```python
from build123d import *

# Parameters (mm, degrees)
BOSS_EXTRUDE1_DEPTH              = 6.35
F_17_64_0_26563_DIAMETER_HOLE1_D = 6.747002
FILLET1_R                        = 6.35
F_10_0_1935_DIAMETER_HOLE1_D     = 4.9149
SKETCH8_R                        = 3.373501
CUT_EXTRUDE1_DEPTH               = 299.268395545
FILLET2_R                        = 12.7


with BuildPart() as part:
    # Sketch1 → Boss-Extrude1 (new body)
    with BuildSketch(Plane(origin=(0, 0, 0), x_dir=(1, 0, 0), z_dir=(0, 1, 0))):
        with BuildLine():
            Line((-268.2875, -15.875), (-233.3625, -15.875))
            ThreePointArc((-233.3625, -15.875), (-228.872371939, -17.734871939), (-227.0125, -22.225))
            Line((-227.0125, -22.225), (-227.0125, -130.175))
            Line((-227.0125, -130.175), (268.2875, -130.175))
            Line((268.2875, -130.175), (268.2875, 130.175))
            Line((268.2875, 130.175), (-268.2875, 130.175))
            Line((-268.2875, 130.175), (-268.2875, -15.875))
        make_face()
    extrude(amount=BOSS_EXTRUDE1_DEPTH)

    # 17/64 (0.26563) Diameter Hole1 (through all)
    with Locations(Plane(origin=(0, 6.35, 0), x_dir=(1, 0, 0), z_dir=(0, 1, 0))):
        with Locations((-246.0625, 104.775), (-246.0625, 3.175), (-220.6625, -53.975), (-220.6625, -117.475), (246.0625, 114.3381), (246.0625, -12.6619)):
            Hole(F_17_64_0_26563_DIAMETER_HOLE1_D / 2)

    # Fillet1
    fillet1_edges = [part.edges().sort_by_distance(p)[0] for p in [
        (268.2875, 3.175, 130.175),
        (-227.0125, 3.175, 130.175),
        (-268.2875, 3.175, 15.875),
        (-268.2875, 3.175, -130.175),
        (268.2875, 3.175, -130.175),
    ]]
    fillet(fillet1_edges, radius=FILLET1_R)

    # #10 (0.1935) Diameter Hole1 (through all)
    with Locations(Plane(origin=(0, 6.35, 0), x_dir=(1, 0, 0), z_dir=(0, 1, 0))):
        with Locations((200.4455889, 98.15353155), (156.73906445, 35.734145775), (113.03254, -26.68524), (100.0125, -53.975), (100.0125, -117.475)):
            Hole(F_10_0_1935_DIAMETER_HOLE1_D / 2)

    # Sketch8 → Cut-Extrude1 (cut, through all)
    with BuildSketch(Plane(origin=(0, 6.35, 0), x_dir=(1, 0, 0), z_dir=(0, 1, 0))):
        with BuildLine():
            Line((-220.6625, -130.175), (87.3125, -130.175))
            Line((87.3125, -130.175), (87.3125, -110.647553384))
            ThreePointArc((87.3125, -110.647553384), (-34.644148174, 53.50332424), (-227.0125, -15.875))
            Line((-227.0125, -15.875), (-233.3625, -15.875))
            ThreePointArc((-233.3625, -15.875), (-228.872371939, -17.734871939), (-227.0125, -22.225))
            Line((-227.0125, -22.225), (-227.0125, -123.825))
            ThreePointArc((-227.0125, -123.825), (-225.152628061, -128.315128061), (-220.6625, -130.175))
        make_face()
        with Locations((-220.6625, -117.475)):
            Circle(SKETCH8_R, mode=Mode.SUBTRACT)
        with Locations((-220.6625, -53.975)):
            Circle(SKETCH8_R, mode=Mode.SUBTRACT)
    extrude(amount=-CUT_EXTRUDE1_DEPTH, mode=Mode.SUBTRACT)

    # Fillet2
    fillet2_edges = [part.edges().sort_by_distance(p)[0] for p in [
        (-227.0125, 3.175, 15.875),
        (87.3125, 3.175, 130.175),
    ]]
    fillet(fillet2_edges, radius=FILLET2_R)


solid = part.part
```
Build history of the part. All positions in model axes, mm. Give positions to 0.01 mm unless a question says otherwise; leave off trailing zeros. Loops run counter-clockwise (first coordinate to the right, second up) from the corner with the lowest first, then second, coordinate; pieces in that order, holes last.
Item 1: Flat gauge pins, fed straight in: pin 1 (4 mm diameter, centred on x = 156.74, z = -35.73, fed in from -Y); pin 2 (3 mm diameter, centred on y = 3.5, z = 114, fed in from -X); pin 3 (1.9 mm diameter, centred on x = -251, y = 3, fed in from +Z) (3 decimals). Where does each tip first touch, or does it go through?
Answers follow:
pin 1: passes through
pin 2: stops at x = 87.31
pin 3: stops at z = 15.875
Item 2: Slice it at D-D, the plane z = 75.5. List the corners of the cut face in (x, y), and give its area (3 significant figures).
Answers follow:
outline: (83.67, 0) - (268.29, 0) - (268.29, 6.35) - (83.67, 6.35) - close
area: 1,170 mm2
Item 3: Slice it at B-B, the plane y = 4.25. Give the number of separate pieces and of enclosed holes in the cut face, and give its area (3 significant figures).
Answers follow:
separate pieces: 1
enclosed holes: 9
area: 84,200 mm2
Item 4: Drill centre lines: line 1 (X direction, y = 2.25, z = -1.5); line 2 (X direction, y = 1, z = -18); line 3 (X direction, y = 2.5, z = 14.5). Where is each one in solid material? Low to high.
Answers follow:
line 1: x = -268.29 to -248.99, -243.13 to -213.82, 45.55 to 268.29
line 2: x = -268.29 to -197.47, 29.2 to 268.29
line 3: x = -265.88 to -227.93, 57.82 to 243.23, 248.89 to 268.29
Item 5: Slice it at C-C, the plane x = -178.5. List the corners of the cut face in (y, z) (3 decimals).
Answers follow:
outline: (0, -130.175) - (6.35, -130.175) - (6.35, -32.499) - (0, -32.499) - close
Item 6: Slice it at A-A, the plane z = -46. List the corners of the cut face in (x, y).
Answers follow:
outline: (-268.29, 0) - (-153.83, 0) - (-153.83, 6.35) - (-268.29, 6.35) - close; (-14.45, 0) - (268.29, 0) - (268.29, 6.35) - (-14.45, 6.35) - close
Item 7: Pull direction X, two halves, no side cores. Call faces 1 (the face through (90.934, 3.131, 126.356)), 2 (the face through (-28.708, 3.219, -51.595)), 3 (the face through (56, 0, -31)): released by +X, released by -X, zero draft, split by the parting line, or undercut.
Answers follow:
face 1: released by -X
face 2: undercut
face 3: zero draft
